from build123d import *

# Parameters (mm, degrees)
SKETCH1_R              = 1.25
SKETCH1_R_2            = 1.5
MAIN_DEPTH             = 3
SKETCH2_W              = 20
SKETCH2_H              = 2
PINHOLES_DEPTH         = 1.5
SKETCH3_W              = 1
SKETCH3_H              = 2.9
MAKERBEAMSUPPORT_DEPTH = 30
SKETCH4_R              = 1.25
SKETCH4_R_2            = 1.5
HOLES2_DEPTH           = 5


with BuildPart() as part:
    # Sketch1 → Main (new body)
    with BuildSketch(Plane.XY):
        Polygon((-10, -7.5), (10, -7.5), (10, -2.5), (20, -2.5), (20, 7.5), (-10, 7.5), align=None)
        with Locations((-7.375, 4.5)):
            Circle(SKETCH1_R, mode=Mode.SUBTRACT)
        with Locations((7.375, 4.5)):
            Circle(SKETCH1_R, mode=Mode.SUBTRACT)
        with Locations((15, 2.5)):
            Circle(SKETCH1_R_2, mode=Mode.SUBTRACT)
    extrude(amount=MAIN_DEPTH)

    # Sketch2 → PinHoles (cut)
    with BuildSketch(Plane.XY.offset(3)):
        with Locations((0, -6.5)):
            Rectangle(SKETCH2_W, SKETCH2_H)
    extrude(amount=-PINHOLES_DEPTH, mode=Mode.SUBTRACT)

    # Sketch3 → MakerBeamSupport (add)
    with BuildSketch(Plane.ZY.offset(10)):
        with Locations((-0.5, 2.5)):
            Rectangle(SKETCH3_W, SKETCH3_H)
    extrude(amount=-MAKERBEAMSUPPORT_DEPTH)

    # Sketch4 → Holes2 (cut, through all)
    with BuildSketch(Plane.XY.offset(3)):
        with Locations((-7.375, 4.5)):
            Circle(SKETCH4_R)
        with Locations((7.375, 4.5)):
            Circle(SKETCH4_R)
        with Locations((15, 2.5)):
            Circle(SKETCH4_R_2)
    extrude(amount=-HOLES2_DEPTH, mode=Mode.SUBTRACT)


solid = part.part
Geometry: final body of the model. Coordinates: model frame, mm. A direction names the side the tool comes from. Give positions to 0.01 mm unless a question says otherwise; leave off trailing zeros. Loops run counter-clockwise (first coordinate to the right, second up) from the corner with the lowest first, then second, coordinate; pieces in that order, holes last. Notation, with made-up numbers: M -2,80.25 L 18,80.25 A15 cw 18,100.25 Z; hole C -12.5,37.25 d4. An arc over 180 degrees is marked long. Put each result on its own line as item: value. Start each with the question number.
1) Cut plane B-B (x = 15). Output: boundary loops of the cut face in (y, z).
2) Cut plane C-C (y = 4.5). Output: boundary loops of the cut face in (x, z) (3 decimals).
3) Access query for faces 4 (the flat face through (5, 6, 0)), 5 (the flat face through (2.1, 1.05, -0.5)), 6 (the flat face through (10, -4, 1)). Directions: +Z, -Z, +X, -X, +Y, -Y. A direction counts if a zero-diameter tool reaches every point of the face in a straight line with its end or side. Return the directions, or none.
4) Cut plane D-D (z = 1.85). Output: boundary loops of the cut face in (x, y) (3 decimals), then the cut area to 3 significant figures.
5) Pull-direction query (Y, two-part tool) for faces 1 (the flat face through (17.7, 1.05, -0.5)), 2 (the flat face through (0, -6, 1.5)), 3 (the cylindrical face through (16.386, 1.925, 1.028)); classes: pulls with the +Y half, pulls with the -Y half, needs draft (parallel to the pull), parting line crosses it, or undercut.
6) Ray query, line 1 along X through (y, z) = (4.5, 0.05) (3 decimals); line 2 along X through (y, z) = (5.5, 1.2) (3 decimals); line 3 along Z through (x, y) = (17.5, -0.5). Return the intervals inside material, ascending.
7) Contact query for flat-ended pins moving along their axis: pin 1 (1.1 mm diameter, centred on x = 0, z = -0.5, fed in from -Y); pin 2 (0.9 mm diameter, centred on y = -4.5, z = 2, fed in from +X); pin 3 (0.8 mm diameter, centred on x = 16.5, z = -0.5, fed in from +Y); pin 4 (3 mm diameter, centred on x = 2, y = -3, fed in from -Z). Output: stop coordinate, or through.
8) Cut plane A-A (y = 2.5). Output: boundary loops of the cut face in (x, z).
Verdict:
1. outline: M -2.5,0 L 1,0 L 1,3 L -2.5,3 Z; M 4,0 L 7.5,0 L 7.5,3 L 4,3 Z
2. outline: M -10,0 L -8.625,0 L -8.625,3 L -10,3 Z; M -6.125,0 L 6.125,0 L 6.125,3 L -6.125,3 Z; M 8.625,0 L 20,0 L 20,3 L 8.625,3 Z
3. face 4: -Z, +X, -X, +Y
3. face 5: -Z, +X, -X, -Y
3. face 6: +Z, -Z, +X, -Y
4. outline: M -10,-5.5 L 10,-5.5 L 10,-2.5 L 20,-2.5 L 20,7.5 L -10,7.5 Z; hole C -7.375,4.5 d2.5; hole C 7.375,4.5 d2.5; hole C 15,2.5 d3
4. area: 343 mm2
5. face 1: pulls with the -Y half
5. face 2: needs draft
5. face 3: undercut
6. line 1: -10 to -8.625, -6.125 to 6.125, 8.625 to 20
6. line 2: -10 to -8.125, -6.625 to 6.625, 8.125 to 20
6. line 3: 0 to 3
7. pin 1: y = -7.5
7. pin 2: x = 10
7. pin 3: y = 3.95
7. pin 4: z = 0
8. outline: M -10,-1 L 13.5,-1 L 13.5,3 L -10,3 Z; M 16.5,-1 L 20,-1 L 20,3 L 16.5,3 Z
